For this review, take the finished solid that the model builds, in its own axes (mm). Face numbers are marked on the shaded views. A direction names the side the tool comes from. Give positions to 0.01 mm unless a question says otherwise; leave off trailing zeros. Write each loop counter-clockwise with the first axis right and the second up, starting at its lowest first coordinate (ties: lowest second). Pieces come first, ordered by that corner, then holes. Notation, with made-up numbers: M 32.5,36.5 L 56.5,36.5 A10 ccw 56.5,55.5 Z; hole C 55,43 d1. An arc over 180 degrees is marked long. One line per item, written item: value. Start each with the question number.
Item 1: Consider section D-D, the plane x = -19. Write out the cut boundary in (y, z), and give its area (3 significant figures).
Item 2: Clearance check with flat-ended pins moving along their axes: pin 1 Ø1 at (x, z) = (-20, -23.5) entering from -Y; pin 2 Ø5.5 at (x, y) = (-31.5, 10) entering from +Z; pin 3 Ø4.5 at (x, z) = (-32.1, -10.43) entering from +Y; pin 4 Ø4 at (x, z) = (25, 12) entering from +Y. State where each tip first meets the part, or that it passes through.
Item 3: Consider section A-A, the plane y = 15. Write out the cut boundary in (x, z).
Item 4: Consider section B-B, the plane x = -11. Write out the cut boundary in (y, z), and give its area (3 significant figures).
Item 5: Tool access review of the marked faces 1 and 2: name each direction out of +Z, -Z, +X, -X, +Y, -Y from which nothing blocks a thin tool from reaching the whole face with its end or side.
Item 6: Mouldability with a two-part tool opening along X and no side actions: class the marked faces 3, 4 and 5 as released by +X, released by -X, zero draft, split by the parting line, or undercut.
Item 7: Consider section C-C, the plane z = 33.75. Write out the cut boundary in (x, y).
Item 8: To check wall thickness, follow probe 1 along X at (y, z) = (11.5, 0); probe 2 along Z at (x, y) = (33, 5.75); probe 3 along Z at (x, y) = (-30.5, 15). State the ranges of each line that lie inside material, in increasing order.
```python
from build123d import *

# Parameters (mm, degrees)
SKETCH1_R                                           = 39
BOSS_EXTRUDE1_DEPTH                                 = 7
SKETCH3_R                                           = 17.5
BOSS_EXTRUDE2_DEPTH                                 = 1
SKETCH4_R                                           = 15
BOSS_EXTRUDE3_DEPTH                                 = 14
SKETCH5_R                                           = 6.25
SKETCH5_R_2                                         = 1.8
CUT_EXTRUDE1_DEPTH                                  = 23
CSK_FOR_M4_COUNTERSUNK_FLAT_HEAD_SCREW1_D           = 3.5
CSK_FOR_M4_COUNTERSUNK_FLAT_HEAD_SCREW1_CSINK_D     = 9.1
CSK_FOR_M4_COUNTERSUNK_FLAT_HEAD_SCREW1_CSINK_ANGLE = 90
SKETCH7_R                                           = 28.5
SKETCH7_R_2                                         = 26.5
BOSS_EXTRUDE4_DEPTH                                 = 10.5
SKETCH8_R                                           = 26.5
SKETCH8_R_2                                         = 17.5
CUT_EXTRUDE2_DEPTH                                  = 1
SKETCH9_R                                           = 2.05
CUT_EXTRUDE3_DEPTH                                  = 8.0000001
BOSS_EXTRUDE5_DEPTH                                 = 10.5
CUT_EXTRUDE4_DEPTH                                  = 8.0000001
FILLET1_R                                           = 1


with BuildPart() as part:
    # Sketch1 → Boss-Extrude1 (new body)
    with BuildSketch(Plane(origin=(0, 0, 0), x_dir=(1, 0, 0), z_dir=(0, 1, 0))):
        Circle(SKETCH1_R)
    extrude(amount=BOSS_EXTRUDE1_DEPTH)

    # Sketch3 → Boss-Extrude2 (add)
    with BuildSketch(Plane(origin=(0, 7, 0), x_dir=(1, 0, 0), z_dir=(0, 1, 0))):
        Circle(SKETCH3_R)
    extrude(amount=BOSS_EXTRUDE2_DEPTH)

    # Sketch4 → Boss-Extrude3 (add)
    with BuildSketch(Plane(origin=(0, 8, 0), x_dir=(1, 0, 0), z_dir=(0, 1, 0))):
        Circle(SKETCH4_R)
    extrude(amount=BOSS_EXTRUDE3_DEPTH)

    # Sketch5 → Cut-Extrude1 (cut, through all)
    with BuildSketch(Plane(origin=(0, 22, 0), x_dir=(1, 0, 0), z_dir=(0, 1, 0))):
        Circle(SKETCH5_R)
        with Locations((0, 11)):
            Circle(SKETCH5_R_2)
        with Locations((11, 0)):
            Circle(SKETCH5_R_2)
        with Locations((0, -11)):
            Circle(SKETCH5_R_2)
        with Locations((-11, 0)):
            Circle(SKETCH5_R_2)
    extrude(amount=-CUT_EXTRUDE1_DEPTH, mode=Mode.SUBTRACT)

    # CSK for M4 Countersunk Flat Head Screw1 (through all)
    with Locations(Plane(origin=(11, 0, 0), x_dir=(0, 0, -1), z_dir=(0, -1, 0))):
        with Locations((0, 0), (11, -11), (0, -22), (-11, -11)):
            CounterSinkHole(CSK_FOR_M4_COUNTERSUNK_FLAT_HEAD_SCREW1_D / 2, CSK_FOR_M4_COUNTERSUNK_FLAT_HEAD_SCREW1_CSINK_D / 2, counter_sink_angle=CSK_FOR_M4_COUNTERSUNK_FLAT_HEAD_SCREW1_CSINK_ANGLE)

    # Sketch7 → Boss-Extrude4 (add)
    with BuildSketch(Plane(origin=(0, 7, 0), x_dir=(1, 0, 0), z_dir=(0, 1, 0))):
        Circle(SKETCH7_R)
        Circle(SKETCH7_R_2, mode=Mode.SUBTRACT)
    extrude(amount=BOSS_EXTRUDE4_DEPTH)

    # Sketch8 → Cut-Extrude2 (cut)
    with BuildSketch(Plane(origin=(0, 7, 0), x_dir=(1, 0, 0), z_dir=(0, 1, 0))):
        Circle(SKETCH8_R)
        Circle(SKETCH8_R_2, mode=Mode.SUBTRACT)
    extrude(amount=-CUT_EXTRUDE2_DEPTH, mode=Mode.SUBTRACT)

    # Sketch9 → Cut-Extrude3 (cut, through all)
    with BuildSketch(Plane(origin=(0, 7, 0), x_dir=(1, 0, 0), z_dir=(0, 1, 0))):
        with Locations((0, 33.75)):
            Circle(SKETCH9_R)
        with Locations((19.837752265, 27.30432356)):
            Circle(SKETCH9_R)
        with Locations((32.098157425, 10.42932356)):
            Circle(SKETCH9_R)
        with Locations((32.098157425, -10.42932356)):
            Circle(SKETCH9_R)
        with Locations((19.837752265, -27.30432356)):
            Circle(SKETCH9_R)
        with Locations((0, -33.75)):
            Circle(SKETCH9_R)
        with Locations((-19.837752265, -27.30432356)):
            Circle(SKETCH9_R)
        with Locations((-32.098157425, -10.42932356)):
            Circle(SKETCH9_R)
        with Locations((-32.098157425, 10.42932356)):
            Circle(SKETCH9_R)
        with Locations((-19.837752265, 27.30432356)):
            Circle(SKETCH9_R)
    extrude(amount=-CUT_EXTRUDE3_DEPTH, mode=Mode.SUBTRACT)

    # Sketch10 → Boss-Extrude5 (add)
    with BuildSketch(Plane(origin=(0, 7, 0), x_dir=(1, 0, 0), z_dir=(0, 1, 0))):
        with BuildLine():
            Line((-33.5, 3), (-28.341665442, 3))
            ThreePointArc((-28.341665442, 3), (-28.5, 0), (-28.341665442, -3))
            Line((-28.341665442, -3), (-33.5, -3))
            ThreePointArc((-33.5, -3), (-36.5, 0), (-33.5, 3))
        make_face()
    extrude(amount=BOSS_EXTRUDE5_DEPTH)

    # Sketch11 → Cut-Extrude4 (cut, through all)
    with BuildSketch(Plane(origin=(0, 7, 0), x_dir=(1, 0, 0), z_dir=(0, 1, 0))):
        with BuildLine():
            Line((35, 4.55), (38.73367398, 4.55))
            ThreePointArc((38.73367398, 4.55), (39, 0), (38.73367398, -4.55))
            Line((38.73367398, -4.55), (35, -4.55))
            ThreePointArc((35, -4.55), (30.45, 0), (35, 4.55))
        make_face()
    extrude(amount=-CUT_EXTRUDE4_DEPTH, mode=Mode.SUBTRACT)

    # Fillet1
    fillet1_edges = [part.edges().sort_by_distance(p)[0] for p in [
        (38.73367398, 3.5, -4.55),
        (38.73367398, 3.5, 4.55),
    ]]
    fillet(fillet1_edges, radius=FILLET1_R)


solid = part.part
```
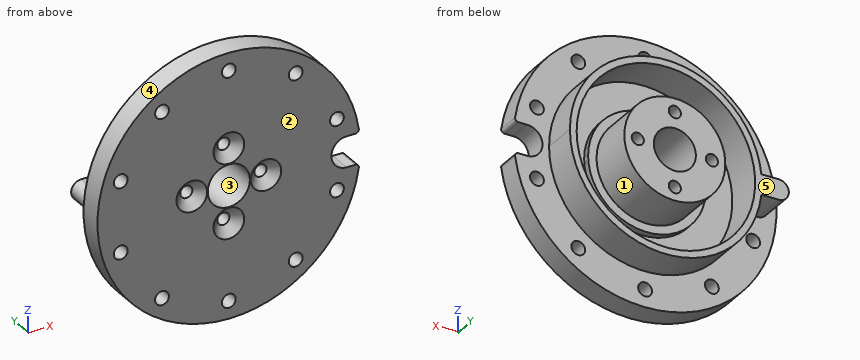
Model answer:
1. outline: M 0,-34.06 L 7,-34.06 L 7,-29.18 L 0,-29.18 Z; M 0,-25.43 L 7,-25.43 L 7,-21.24 L 17.5,-21.24 L 17.5,-18.47 L 6,-18.47 L 6,18.47 L 17.5,18.47 L 17.5,21.24 L 7,21.24 L 7,25.43 L 0,25.43 Z; M 0,29.18 L 7,29.18 L 7,34.06 L 0,34.06 Z
1. area: 446 mm2
2. pin 1: stops at y = 0
2. pin 2: stops at z = 3
2. pin 3: stops at y = 7
2. pin 4: stops at y = 17.5
3. outline: M -33.5,-3 L -28.34,-3 A28.5 ccw long -28.34,3 L -33.5,3 A3 ccw Z; C 0,0 d30; hole C 0,0 d53; hole C -11,0 d3.6; hole C 0,0 d12.5; hole C 0,-11 d3.6; hole C 0,11 d3.6; hole C 11,0 d3.6
4. outline: M 0,-37.42 L 7,-37.42 L 7,-26.29 L 17.5,-26.29 L 17.5,-24.11 L 6,-24.11 L 6,-13.61 L 8,-13.61 L 8,-10.2 L 22,-10.2 L 22,-1.8 L 2.75,-1.8 L 0,-4.55 Z; M 0,4.55 L 2.75,1.8 L 22,1.8 L 22,10.2 L 8,10.2 L 8,13.61 L 6,13.61 L 6,24.11 L 17.5,24.11 L 17.5,26.29 L 7,26.29 L 7,37.42 L 0,37.42 Z
4. area: 775 mm2
5. face 1: +Y
5. face 2: +Z, -Z, +X, -X, -Y
6. face 3: undercut
6. face 4: split by the parting line
6. face 5: zero draft
7. outline: M -19.54,0 L -2.05,0 L -2.05,7 L -19.54,7 Z; M 2.05,0 L 19.54,0 L 19.54,7 L 2.05,7 Z
8. probe 1: x = -36.5 to -26.5, -15 to -12.8, -9.2 to -6.25, 6.25 to 9.2, 12.8 to 15, 26.5 to 28.5
8. probe 2: z = -20.78 to -12.27, -8.59 to -4.09, 4.09 to 8.59, 12.27 to 20.78
8. probe 3: z = -3 to 3
